Autodesk Inventor part; units mm, degrees
ref_plane "Work Plane1" through (0, 3.81, 0) normal (0, 1, 0) x (1, 0, 0)
ref_plane "YZ Plane" through (0, 0, 0) normal (1, 0, 0) x (0, 1, 0)
ref_plane "XZ Plane" through (0, 0, 0) normal (0, 1, 0) x (-1, 0, 0)
sketch "Sketch1" plane through (0, 0, 0) normal (0, 0, 1) x (1, 0, 0)
  line L0 (0, 0) -> (0, 8.6646) construction
  line L1 (20.9931, 1.27) -> (20.9931, 5.715)
  line L2 (20.9931, 5.715) -> (27.9781, 3.81)
  line L3 (27.9781, 3.81) -> (27.9781, 0)
  line L4 (27.9781, 0) -> (20.9931, 0)
  line L5 (20.9931, 1.27) -> (18.4531, 1.27)
  line L6 (18.4531, 1.27) -> (18.4531, 0)
  line L7 (18.4531, 0) -> (20.9931, 0)
  dimension "d0" = 20.9931
  dimension "d1" = 4.445
  dimension "d2" = 1.27
  dimension "d3" = 2.54
  dimension "d4" = 3.81
  dimension "d5" = 6.985
revolve "Revolution1" add sketch "Sketch1" angle 360 about axis through (0, 0, 0) along (0, 1, 0)
ref_plane "Work Plane1" through (0, 3.81, 0) normal (0, 1, 0) x (1, 0, 0)
sketch "Sketch2" plane through (0, 0, 0) normal (0, -1, 0) x (1, 0, 0)
  line L0 (0, 0) -> (-45.8206, 0) construction
  circle A0 centre (0, 0) radius 27.9781
  line L1 (-27.6227, 4.445) -> (-30.5181, 2.54)
  line L2 (-30.5181, 2.54) -> (-30.5181, -2.54)
  line L3 (-30.5181, -2.54) -> (-27.6227, -4.445)
  dimension "d7" = 2.54
  dimension "d8" = 8.89
  dimension "d9" = 5.08
extrude "Extrusion1" add sketch "Sketch2" against normal up to surface (3.81 mm away) contours A0 L3 L2 L1
pattern_circular "Circular Pattern1" count 12 over 360 about axis through (0, 1.905, 0) along (0, -1, 0) of "Extrusion1"
sketch "Sketch4" plane through (0, 1.27, 0) normal (0, 1, 0) x (1, 0, 0)
  circle A0 centre (0, 0) radius 20.9931
  arc A1 (-26.1445, 9.9619) -> (-27.6227, 4.445) centre (0, 0) ccw
  arc A2 (-27.6227, 4.445) -> (-27.6227, -4.445) centre (0, 0) ccw
  arc A3 (-27.6227, -4.445) -> (-26.1445, -9.9619) centre (0, 0) ccw
  arc A4 (-26.1445, -9.9619) -> (-21.6995, -17.6609) centre (0, 0) ccw
  arc A5 (-21.6995, -17.6609) -> (-17.6609, -21.6995) centre (0, 0) ccw
  arc A6 (-17.6609, -21.6995) -> (-9.9619, -26.1445) centre (0, 0) ccw
  arc A7 (-9.9619, -26.1445) -> (-4.445, -27.6227) centre (0, 0) ccw
  arc A8 (-4.445, -27.6227) -> (4.445, -27.6227) centre (0, 0) ccw
  arc A9 (4.445, -27.6227) -> (9.9619, -26.1445) centre (0, 0) ccw
  arc A10 (9.9619, -26.1445) -> (17.6609, -21.6995) centre (0, 0) ccw
  arc A11 (17.6609, -21.6995) -> (21.6995, -17.6609) centre (0, 0) ccw
  arc A12 (21.6995, -17.6609) -> (26.1445, -9.9619) centre (0, 0) ccw
  arc A13 (26.1445, -9.9619) -> (27.6227, -4.445) centre (0, 0) ccw
  arc A14 (27.6227, -4.445) -> (27.6227, 4.445) centre (0, 0) ccw
  arc A15 (27.6227, 4.445) -> (26.1445, 9.9619) centre (0, 0) ccw
  arc A16 (26.1445, 9.9619) -> (21.6995, 17.6609) centre (0, 0) ccw
  arc A17 (21.6995, 17.6609) -> (17.6609, 21.6995) centre (0, 0) ccw
  arc A18 (17.6609, 21.6995) -> (9.9619, 26.1445) centre (0, 0) ccw
  arc A19 (9.9619, 26.1445) -> (4.445, 27.6227) centre (0, 0) ccw
  arc A20 (4.445, 27.6227) -> (-4.445, 27.6227) centre (0, 0) ccw
  arc A21 (-4.445, 27.6227) -> (-9.9619, 26.1445) centre (0, 0) ccw
  arc A22 (-9.9619, 26.1445) -> (-17.6609, 21.6995) centre (0, 0) ccw
  arc A23 (-17.6609, 21.6995) -> (-21.6995, 17.6609) centre (0, 0) ccw
  arc A24 (-21.6995, 17.6609) -> (-26.1445, 9.9619) centre (0, 0) ccw
  circle A25 centre (0, 0) radius 18.4531
  circle A26 centre (0, 0) radius 20.9931
  circle A27 centre (24.1681, -3.81) radius 1.27
  circle A28 centre (24.1681, -3.81) radius 0.635
  line L0 (30.5181, 2.54) -> (30.5181, -2.54)
  arc A29 (17.9659, -17.8891) -> (17.3155, -16.3716) centre (19.0881, -16.51) ccw
  line L1 (19.0881, -16.51) -> (15.2571, -18.1519) construction
  line L2 (18.7629, -15.7512) -> (17.3155, -16.3716)
  line L3 (17.9659, -17.8891) -> (19.4133, -17.2688)
  arc A30 (19.4133, -17.2688) -> (18.7629, -15.7512) centre (19.0881, -16.51) ccw
  line L4 (19.0881, -16.51) -> (24.1681, -3.81) construction
  line L5 (19.1153, -14.7322) -> (23.17, -4.5954)
  line L6 (20.2945, -15.2039) -> (24.3492, -5.067)
  point P0 (17.1726, -17.3309)
  dimension "d19" = 2.54
  dimension "d20" = 0.635
  dimension "d22" = 3.81
  dimension "d23" = 6.35
  dimension "d24" = 3.556
  dimension "d25" = 135
  dimension "d26" = 1.27
  dimension "d27" = 0.635
  dimension "d28" = 12.7
  dimension "d29" = 5.08
  dimension "d30" = 1.651
extrude "Extrusion3" cut sketch "Sketch4" along normal through all contours A27 | A27 L6 A29 L5 | A29 L3 A30 L2
fillet "Fillet1" radius 3.175 4 edges at (19.1153, 3.0642, 14.7322) (20.2945, 2.8973, 15.2039) (23.17, 3.1341, 4.5954) (24.3492, 2.9637, 5.067)
pattern_circular "Circular Pattern2" count 3 over 90 about axis through (0, 3.4925, 0) along (0, -1, 0) of "Extrusion3", "Fillet1"
mirror "Mirror1" about plane through (0, 0, 0) normal (0, 0, 1) of "Extrusion3", "Fillet1", "Circular Pattern2"
sketch "Sketch5" plane through (0, 1.27, 0) normal (0, 1, 0) x (1, 0, 0)
  line L0 (0, 0) -> (-35.8156, 0)
  line L1 (-35.8156, 0) -> (-35.8156, -45.2748)
  line L2 (-35.8156, -45.2748) -> (0, -45.2748)
  line L3 (0, -45.2748) -> (0, 0)
extrude "Extrusion4" cut sketch "Sketch5" along normal through all both and the other way through all keep common part
sketch "Sketch6" plane through (-2.54, 0, 30.5181) normal (0, -1, 0) x (1, 0, 0)
  line L0 (2.54, -9.525) -> (2.54, -2.54)
  arc A0 (2.54, -9.525) -> (-18.4531, -30.5181) centre (2.54, -30.5181) ccw
  line L1 (-25.4381, -30.5181) -> (-18.4531, -30.5181)
  arc A1 (-25.0827, -26.0731) -> (-25.4381, -30.5181) centre (2.54, -30.5181) ccw
  arc A2 (-23.6045, -20.5562) -> (-25.0827, -26.0731) centre (2.54, -30.5181) ccw
  arc A3 (-19.1595, -12.8572) -> (-23.6045, -20.5562) centre (2.54, -30.5181) ccw
  arc A4 (-15.1209, -8.8186) -> (-19.1595, -12.8572) centre (2.54, -30.5181) ccw
  arc A5 (-7.4219, -4.3736) -> (-15.1209, -8.8186) centre (2.54, -30.5181) ccw
  arc A6 (-1.905, -2.8954) -> (-7.4219, -4.3736) centre (2.54, -30.5181) ccw
  arc A7 (2.54, -2.54) -> (-1.905, -2.8954) centre (2.54, -30.5181) ccw
  line L2 (-3.6316, -6.6107) -> (-11.2674, -9.665)
  line L3 (-15.3491, -12.5522) -> (-14.7288, -11.1048)
  line L4 (-13.2112, -11.7552) -> (-13.8316, -13.2026)
  line L5 (-10.7957, -10.8442) -> (-3.1599, -7.7899)
  arc A8 (-23.6045, -20.5562) -> (-25.0827, -26.0731) centre (2.54, -30.5181) ccw
  line L6 (-25.0827, -26.0731) -> (-30.8234, -26.6683)
  line L7 (-30.8234, -26.6683) -> (-31.3133, -31.1273)
  line L8 (-31.3133, -31.1273) -> (-25.4381, -30.5181)
  line L9 (2.54, -2.54) -> (2.54, 0)
  arc A9 (2.54, -2.54) -> (-1.905, -2.8954) centre (2.54, -30.5181) ccw
  arc A10 (2.54, -2.54) -> (-1.905, -2.8954) centre (2.54, -30.5181) ccw
  line L10 (-1.905, -2.8954) -> (-3.1599, 4.5152)
  line L11 (-3.1599, 4.5152) -> (4.4262, 3.6816)
  line L12 (4.4262, 3.6816) -> (2.54, -2.54)
  point P0 (-2.2816, -5.5822)
  point P1 (-13.4231, -9.7382)
  point P2 (-12.4072, -12.2779)
  point P3 (-1.4731, -7.6037)
extrude "Extrusion5" cut sketch "Sketch6" along normal through all both and the other way through all contours A7 L10 L11 L12 | L8 L7 L6 A1
sketch "Sketch7" plane through (-20.9931, 1.27, 0) normal (0, 1, 0) x (1, 0, 0)
  point P0 (20.9931, 0)
equation "\"d27\" = 0.5 * d26"
properties part number "Mentor-Mechanical ring"
Geometry check sheet. Reference: the model listing, model coordinates, mm. A direction names the side the tool comes from. Round coordinates to 2 decimals unless told otherwise and drop trailing zeros. Order: outer loops, then holes, each group sorted by start corner. A loop starts at its lowest first (then second) coordinate and runs counter-clockwise, first axis right, second up. Notation, with made-up numbers: M -13.75,-9.75 L 4.25,-9.75 A4 ccw 4.25,-2.75 Z; hole C -15.5,42.5 d7. An arc over 180 degrees is marked long. Answer in a Markdown table with one row per item. Add a question column.
Item 1: Material ranges on L1, parallel to Z at x = -3.81, y = 2.7; L2, parallel to Y at x = -12.75, z = 21; L3, parallel to Z at x = -3.25, y = 3.3, recorded low to high. Write a range as [from, to].
Item 2: Set-up check for faces 5 (the face through (-25, 3.81, 15)), 6 (the face through (-14.86, 2.97, 20.63)), 7 (the face through (-23, 2, 0)): record each of +Z, -Z, +X, -X, +Y, -Y from which the full face is reachable in a straight line by a thin tool's end or side.
Item 3: Depth check by flat-ended pin: pin 1 Ø10.5 at (x, z) = (-7, 12) entering from +Y; pin 2 Ø1.8 at (x, z) = (-14, 23.5) entering from +Y; pin 3 Ø1 at (x, y) = (-6.5, 3.5) entering from +Z. Enter the tip coordinate at first touch or a pass-through.
Item 4: Sectioned sample at A-A, the plane y = 0.5. Enter the section's corners in (x, z) (1 decimal).
Item 5: Draft check along Z on faces 1 (the face through (-15.55, 3.13, 17.59)), 2 (the face through (-14, 1.27, 13)), 3 (the face through (-7.203, 1.878, 27.035)), 4 (the face through (-10.04, 2.99, 22.36)). Enter one of: released by +Z, released by -Z, zero draft, split by the parting line, or undercut.
Filled in:
| question | item | result |
|---|---|---|
| 1 | L1 | z = [20.64, 22.9], [23.53, 24.8], [25.44, 27.72] |
| 1 | L2 | y = [0, 1.27] |
| 1 | L3 | z = [20.74, 23.03], [23.87, 24.47], [25.31, 27.79] |
| 2 | face 5 | +Z, -X, +Y |
| 2 | face 6 | +Y |
| 2 | face 7 | -Z, +X, -X, +Y, -Y |
| 3 | pin 1 | stops at y = 1.27 |
| 3 | pin 2 | stops at y = 4.23 |
| 3 | pin 3 | stops at z = 27.33 |
| 4 | outline | M -28,0 L -18.5,0 A18.5 cw 0,18.5 L 0,28 A28 ccw -4.4,27.6 A28 ccw -10,26.1 L -13.1,27.7 L -17.5,25.2 L -17.7,21.7 A28 ccw -21.7,17.7 L -25.2,17.5 L -27.7,13.1 L -26.1,10 A28 ccw -27.6,4.4 A28 ccw Z |
| 5 | face 1 | undercut |
| 5 | face 2 | zero draft |
| 5 | face 3 | released by +Z |
| 5 | face 4 | undercut |
